Check sheet for the drawn part. Datum: minimum x, y, z corner. Units: mm. A direction names the side the tool comes from. Give positions to 0.01 mm unless a question says otherwise; leave off trailing zeros. Order: outer loops, then holes, each group sorted by start corner. A loop starts at its lowest first (then second) coordinate and runs counter-clockwise, first axis right, second up.
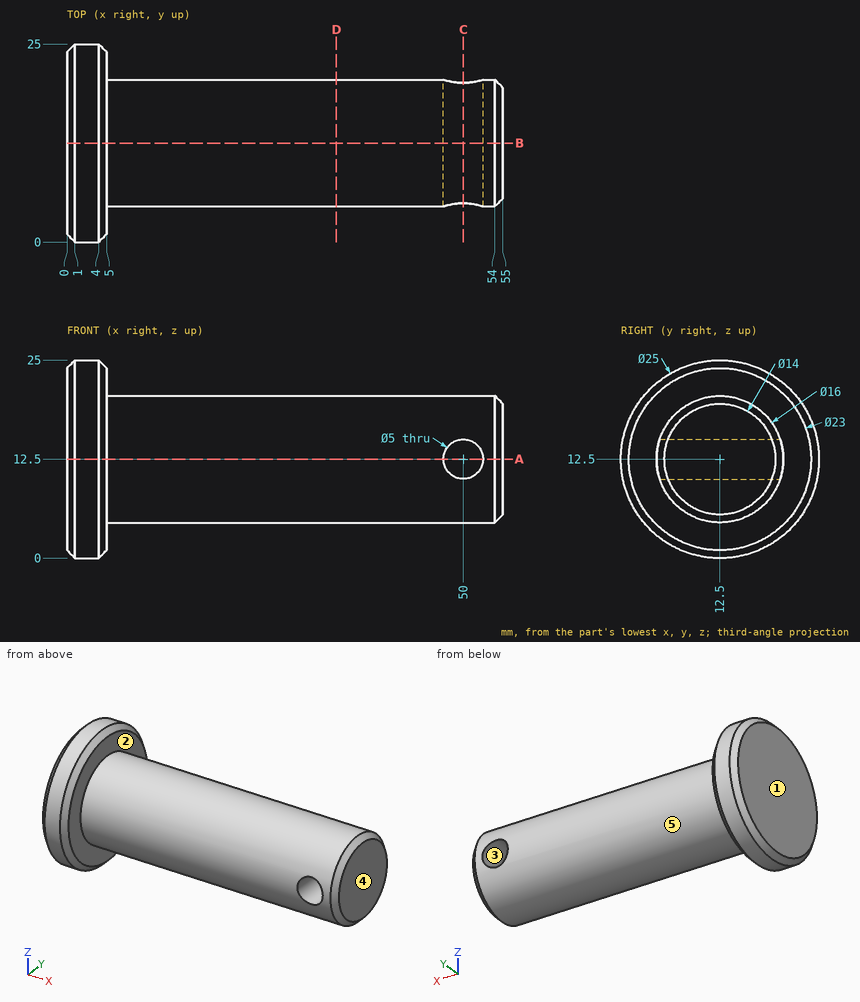
Item 1: Gauge pin test, flat ends, axial feed: pin 1 (8 mm diameter, centred on x = 50, z = 12.5, fed in from +Y); pin 2 (4 mm diameter, centred on x = 9, z = 9, fed in from +Y); pin 3 (3 mm diameter, centred on x = 26, y = 5.5, fed in from -Z). Record the tip position at first contact, or that the pin passes through.
Reported:
pin 1: stops at y = 20.5
pin 2: stops at y = 20.36
pin 3: stops at z = 6.69
Item 2: Sectioned sample at D-D (x = 34). Enter the section's corners in (y, z).
Reported:
outline: circle Ø16 at (12.5, 12.5)
Item 3: Sectioned sample at B-B (y = 12.5). Enter the section's corners in (x, z), and give its area (3 significant figures).
Reported:
outline: (0, 1) - (1, 0) - (4, 0) - (5, 1) - (5, 4.5) - (54, 4.5) - (55, 5.5) - (55, 19.5) - (54, 20.5) - (5, 20.5) - (5, 24) - (4, 25) - (1, 25) - (0, 24) - close; hole circle Ø5 at (50, 12.5)
area: 902 mm2
Item 4: Scan lines: L1, parallel to X at y = 17.75, z = 12.5; L2, parallel to X at y = 17, z = 22.5; L3, parallel to Z at x = 51.5, y = 17. Record each from-to range of solid material in increasing order.
Reported:
L1: x = 0 to 47.5, 52.5 to 55
L2: x = 0 to 5
L3: z = 5.89 to 10.5, 14.5 to 19.11
Item 5: Draft check along Z on the marked faces 3, 4 and 5. Enter one of: released by +Z, released by -Z, zero draft, split by the parting line, or undercut.
Reported:
face 3: undercut
face 4: zero draft
face 5: split by the parting line
Item 6: Sectioned sample at C-C (x = 50). Enter the section's corners in (y, z).
Reported:
outline: (4.9, 10) arc R8 ccw to (20.1, 10) - close; (4.9, 15) - (20.1, 15) arc R8 ccw to start
Item 7: Sectioned sample at A-A (z = 12.5). Enter the section's corners in (x, y).
Reported:
outline: (0, 1) - (1, 0) - (4, 0) - (5, 1) - (5, 4.5) - (47.5, 4.5) - (47.5, 20.5) - (5, 20.5) - (5, 24) - (4, 25) - (1, 25) - (0, 24) - close; (52.5, 4.5) - (54, 4.5) - (55, 5.5) - (55, 19.5) - (54, 20.5) - (52.5, 20.5) - close
Item 8: Set-up check for the marked faces 1 and 2: record each of +Z, -Z, +X, -X, +Y, -Y from which the full face is reachable in a straight line by a thin tool's end or side.
Reported:
face 1: +Z, -Z, -X, +Y, -Y
face 2: +X
